Check sheet for the modelled part. Datum: model origin and axes. Units: mm. A direction names the side the tool comes from. Give positions to 0.01 mm unless a question says otherwise; leave off trailing zeros. Loops run counter-clockwise (first coordinate to the right, second up) from the corner with the lowest first, then second, coordinate; pieces in that order, holes last. Notation, with made-up numbers: M 37.25,82.5 L 90.25,82.5 A4 cw 90.25,88.5 Z; hole C -2.5,37 d2. An arc over 180 degrees is marked long. Write each question's results on one line, items separated by ' | '. Start each with the question number.
1. Draft check along Y on faces 1 (the flat face through (2.75, 18, -17)), 2 (the flat face through (2, 18, -12.5)), 3 (the cylindrical face through (0.6, 79.43, -17.28)). Enter one of: pulls with the +Y half, pulls with the -Y half, needs draft (parallel to the pull), parting line crosses it, or undercut.
2. Tool access check on faces 4 (the cylindrical face through (3.2, 1.2, -22.5)), 5 (the flat face through (6, 0, -18)), 6 (the flat face through (5, 77, -8)). Record the directions out of +Z, -Z, +X, -X, +Y, -Y that give a thin tool (end or side, any length) a straight path to the whole face; none if there is none.
3. Go/stop test with flat-tipped pins: pin 1 (1.8 mm diameter, centred on y = 4, z = -4, fed in from +X); pin 2 (2 mm diameter, centred on y = 0.5, z = -19, fed in from -X); pin 3 (0.8 mm diameter, centred on x = 1.5, z = -15.5, fed in from -Y). Record where each tip stops, or that it passes through.
4. Sectioned sample at C-C on x = 4.25. Give the number of separate pieces and of enclosed holes in the cut face, and give its area (3 significant figures).
5. Material ranges on line 1 along Z through (x, y) = (1.75, 76); line 2 along Y through (x, z) = (4.5, -4); line 3 along Z through (x, y) = (2.25, 28), recorded low to high.
6. Sectioned sample at B-B on y = 17.5. Record the cut outline in (x, z), and give its area (3 significant figures).
7. Sectioned sample at A-A on z = -17.5. Record the cut outline in (x, y).
8. Sectioned sample at D-D on z = -10. Record the cut outline in (x, y).
Autodesk Inventor part; units mm, degrees
ref_plane "YZ Plane" through (0, 0, 0) normal (1, 0, 0) x (0, 1, 0)
ref_plane "XZ Plane" through (0, 0, 0) normal (0, 1, 0) x (-1, 0, 0)
ref_plane "XY Plane" through (0, 0, 0) normal (0, 0, 1) x (1, 0, 0)
sketch "스케치1" plane through (0, 0, 0) normal (1, 0, 0) x (0, 1, 0)
  line L0 (0, 0) -> (80, 0)
  line L1 (80, 0) -> (80, -35)
  line L2 (80, -35) -> (0, -35)
  line L3 (0, -35) -> (0, 0)
  dimension "d0" = 35
  dimension "d1" = 80
extrude "돌출1" add sketch "스케치1" along normal blind 8.75
sketch "스케치2" plane through (8.75, 0, 0) normal (1, 0, 0) x (0, 0, -1)
  line L0 (35, 80) -> (0, 80)
  line L1 (35, 0) -> (35, 80)
  line L2 (0, 80) -> (0, 0)
  line L3 (0, 0) -> (35, 0)
  line L4 (2.5, 77.5) -> (32.5, 77.5)
  line L5 (32.5, 77.5) -> (32.5, 2.5)
  line L6 (32.5, 2.5) -> (2.5, 2.5)
  line L7 (2.5, 2.5) -> (2.5, 77.5)
  dimension "d4" = 2.5
extrude "돌출2" cut sketch "스케치2" against normal blind 7.5 contours L4 L5 L6 L7
sketch "스케치3" plane through (0, 0, -35) normal (0, -1, 0) x (1, 0, 0)
  line L0 (1.25, 22.5) -> (5.25, 22.5)
  line L1 (5.25, 22.5) -> (5.25, 12.5)
  line L2 (5.25, 12.5) -> (1.25, 12.5)
  line L3 (1.25, 12.5) -> (1.25, 22.5)
  line L4 (1.25, 2.5) -> (1.25, 32.5)
  line L5 (0, 0) -> (8.75, 0)
  line L6 (0, 35) -> (8.75, 35)
  circle A0 centre (3.25, 14.5) radius 2
  circle A1 centre (3.25, 20.5) radius 2
  point P0 (1.25, 14.5)
  point P1 (5.25, 14.5)
  point P2 (5.25, 20.5)
  point P3 (1.25, 20.5)
  dimension "d7" = 4
  dimension "d8" = 10
  dimension "d9" = 12.5
  dimension "d10" = 35
extrude "돌출3" cut sketch "스케치3" against normal blind 2.5 contours A1 | A1 L1 A0 L3 | A0
sketch "스케치6" plane through (1.25, 0, 0) normal (1, 0, 0) x (0, 0, -1)
  line L0 (12.5, 14) -> (22.5, 14)
  line L1 (22.5, 14) -> (22.5, 22)
  line L2 (22.5, 22) -> (12.5, 22)
  line L3 (12.5, 22) -> (12.5, 14)
  line L4 (14.5, 0) -> (12.5, 0)
  line L5 (22.5, 0) -> (20.5, 0)
  line L6 (20.5, 0) -> (14.5, 0)
  point P0 (0, 0)
  dimension "d22" = 14
  dimension "d23" = 8
extrude "돌출6" add sketch "스케치6" along normal blind 1.5
sketch "스케치4" plane through (8.75, 0, 0) normal (1, 0, 0) x (0, 0, -1)
  line L0 (35, 0) -> (27, 0)
  line L1 (27, 0) -> (27, 8)
  line L2 (27, 8) -> (35, 8)
  line L3 (35, 8) -> (35, 0)
  line L4 (0, 0) -> (8, 0)
  line L5 (8, 0) -> (8, 8)
  line L6 (8, 8) -> (0, 8)
  line L7 (0, 8) -> (0, 0)
  line L8 (0, 80) -> (8, 80)
  line L9 (8, 80) -> (8, 72)
  line L10 (8, 72) -> (0, 72)
  line L11 (0, 72) -> (0, 80)
  line L12 (35, 0) -> (35, 80)
  line L13 (35, 80) -> (27, 80)
  line L14 (27, 80) -> (27, 72)
  line L15 (27, 72) -> (35, 72)
  line L16 (35, 72) -> (35, 80)
  circle A0 centre (4, 76) radius 4
  circle A1 centre (31, 76) radius 4
  circle A2 centre (31, 4) radius 4
  circle A3 centre (4, 4) radius 4
  circle A4 centre (4, 4) radius 1.5
  circle A5 centre (31, 4) radius 1.5
  circle A6 centre (31, 76) radius 1.5
  circle A7 centre (4, 76) radius 1.5
  point P0 (8, 4)
  point P1 (4, 8)
  point P2 (31, 8)
  point P3 (27, 4)
  point P4 (4, 72)
  point P5 (8, 76)
  point P6 (27, 76)
  point P7 (31, 72)
  dimension "d14" = 8
  dimension "d16" = 3
extrude "돌출4" add sketch "스케치4" against normal up to next contours L0 A2 L3 | L0 L1 A2 | A2 | A2 L2 L3 | L7 A3 L4 | A3 L5 L4 | A3 | L7 L6 A3 | L8 A0 L11 | L8 L9 A0 | A0 | A0 L10 L11 | L15 A1 L12 | A1 L13 L12 | A1 | A1 L14 L13
sketch "스케치7" plane through (0, 80, 0) normal (0, 1, 0) x (1, 0, 0)
  circle A0 centre (5, 17.5) radius 2
  line L0 (0, 35) -> (8.75, 35)
  line L1 (0, 0) -> (8.75, 0)
  line L2 (0, 35) -> (0, 0)
  point P0 (-3.75, 35)
  point P1 (0, 27)
  dimension "d26" = 4
  dimension "d27" = 35
  dimension "d28" = 17.5
  dimension "d29" = 5
extrude "돌출7" cut sketch "스케치7" against normal blind 2.5
fillet "모깎기2" radius 2 8 edges at (4.375, 80, 0) (0, 80, -17.5) (0, 40, -35) (4.375, 0, -35) (0, 0, -17.5) (0, 40, 0) (4.375, 0, 0) (4.375, 80, -35)
equation "\"d9\" = -0.5 * d8 + 0.5 * d10"
equation "\"d28\" = 0.5 * d27"
properties part number "111"
Output values:
1) face 1: needs draft | face 2: undercut | face 3: pulls with the +Y half
2) face 4: -Y | face 5: +Z, -Z, +X, -X, -Y | face 6: +X
3) pin 1: x = 1.25 | pin 2: x = 0.06 | pin 3: y = 0.15
4) separate pieces: 2 | enclosed holes: 4 | area: 593 mm2
5) line 1: -34.98 to -32.5, -29.5 to -27, -8 to -5.5, -2.5 to -0.02 | line 2: 0 to 2.5, 5.5 to 8, 72 to 74.5, 77.5 to 80 | line 3: -35 to -32.5, -2.5 to 0
6) outline: M 0,-33 A2 ccw 2,-35 L 8.75,-35 L 8.75,-32.5 L 1.25,-32.5 L 1.25,-22.5 L 2.75,-22.5 L 2.75,-12.5 L 1.25,-12.5 L 1.25,-2.5 L 8.75,-2.5 L 8.75,0 L 2,0 A2 ccw 0,-2 Z | area: 94.5 mm2
7) outline: M 0,2 A2 ccw 1.25,0.15 L 1.25,14 L 2.75,14 L 2.75,22 L 1.25,22 L 1.25,77.5 L 3,77.5 L 3,80 L 2,80 A2 ccw 0,78 Z; M 5.25,0 L 8.75,0 L 8.75,2.5 L 5.25,2.5 Z; M 7,77.5 L 8.75,77.5 L 8.75,80 L 7,80 Z
8) outline: M 0,2 A2 ccw 2,0 L 8.75,0 L 8.75,2.5 L 1.25,2.5 L 1.25,77.5 L 8.75,77.5 L 8.75,80 L 2,80 A2 ccw 0,78 Z
